Model file for the job. Use its own axes, mm. A direction names the side the tool comes from. Give positions to 0.01 mm unless a question says otherwise; leave off trailing zeros. Loops run counter-clockwise (first coordinate to the right, second up) from the corner with the lowest first, then second, coordinate; pieces in that order, holes last. Notation, with made-up numbers: M 52,36 L 101,36 A32 ccw 101,66 Z; hole C 11,-25 d11. An arc over 180 degrees is marked long. Answer in a Markdown table with one row per item.
Autodesk Inventor part; units mm, degrees
ref_plane "YZ Plane" through (0, 0, 0) normal (1, 0, 0) x (0, 1, 0)
ref_plane "XZ Plane" through (0, 0, 0) normal (0, 1, 0) x (-1, 0, 0)
ref_plane "XY Plane" through (0, 0, 0) normal (0, 0, 1) x (1, 0, 0)
sketch "Sketch1" plane through (0, 0, 0) normal (0, 1, 0) x (-1, 0, 0)
  line L0 (0.5335, -0.6929) -> (33.0335, -0.6929)
  line L1 (33.0335, -0.6929) -> (33.0335, -33.1929)
  line L2 (33.0335, -33.1929) -> (0.5335, -33.1929)
  line L3 (0.5335, -33.1929) -> (0.5335, -0.6929)
  line L4 (-0.7165, 0.5571) -> (34.2835, 0.5571)
  line L5 (34.2835, 0.5571) -> (34.2835, -34.4429)
  line L6 (34.2835, -34.4429) -> (-0.7165, -34.4429)
  line L7 (-0.7165, -34.4429) -> (-0.7165, 0.5571)
  point P0 (0, 0)
  dimension "d0" = 32.5
  dimension "d1" = 32.5
  dimension "d2" = 35
  dimension "d3" = 35
  dimension "d4" = 1.25
  dimension "d5" = 1.25
extrude "Extrusion1" add sketch "Sketch1" along normal blind 3
sketch "Sketch2" plane through (0, 3, 0) normal (0, 1, 0) x (1, 0, 0)
  line L0 (-34.2835, -0.5571) -> (0.7165, -0.5571)
  line L1 (0.7165, -0.5571) -> (0.7165, 34.4429)
  line L2 (-34.2835, -0.5571) -> (0.7165, -0.5571)
  line L3 (0.7165, -0.5571) -> (0.7165, 34.4429)
  line L4 (0.7165, 34.4429) -> (-34.2835, 34.4429)
  line L5 (-34.2835, 34.4429) -> (-34.2835, -0.5571)
  point P0 (0, 0)
extrude "Extrusion2" add sketch "Sketch2" along normal blind 3
sketch "Sketch3" plane through (0, 6, 0) normal (0, 1, 0) x (1, 0, 0)
  line L0 (-21.2835, 12.4429) -> (-12.2835, 12.4429)
  line L1 (-12.2835, 12.4429) -> (-12.2835, 21.4429)
  line L2 (-12.2835, 21.4429) -> (-21.2835, 21.4429)
  line L3 (-21.2835, 21.4429) -> (-21.2835, 12.4429)
  line L4 (-34.2835, 34.4429) -> (-34.2835, -0.5571)
  line L5 (0.7165, 34.4429) -> (-34.2835, 34.4429)
  point P0 (0, 0)
  dimension "d10" = 9
  dimension "d11" = 9
  dimension "d12" = 13
  dimension "d13" = 13
extrude "Extrusion3" cut sketch "Sketch3" against normal blind 3
properties part number "test_camera_seat"
Q1. 3-axis set-ups, long thin cutter, end or side, ignore diameter. For faces 4 (the face through (-17, 5, -21.443)), 5 (the face through (-25, 6, -17)), 6 (the face through (-17, 1, -33.193)): which of +Z, -Z, +X, -X, +Y, -Y reach the whole face in a straight line?
Reported:
| item | result |
|---|---|
| face 4 | +Y, -Y |
| face 5 | +Z, -Z, +X, -X, +Y |
| face 6 | -Y |
Q2. Saw through at D-D (z = -18.5). Give the cut face in (x, y), and give its area (3 significant figures).
Reported:
| item | result |
|---|---|
| outline | M -34.28,0 L -33.03,0 L -33.03,3 L -21.28,3 L -21.28,6 L -34.28,6 Z; M -12.28,3 L -0.53,3 L -0.53,0 L 0.72,0 L 0.72,6 L -12.28,6 Z |
| area | 85.5 mm² |
Q3. Drop a flat-ended pin along its axis: pin 1 (1 mm diameter, centred on x = -23, z = -4, fed in from -Y). Give the stop position or say it passes through.
Reported:
| item | result |
|---|---|
| pin 1 | y = 3 |
Q4. Saw through at A-A (x = -13.5). Give the cut face in (y, z), and give its area (3 significant figures).
Reported:
| item | result |
|---|---|
| outline | M 0,-34.44 L 6,-34.44 L 6,-21.44 L 3,-21.44 L 3,-33.19 L 0,-33.19 Z; M 0,-0.69 L 3,-0.69 L 3,-12.44 L 6,-12.44 L 6,0.56 L 0,0.56 Z |
| area | 85.5 mm² |
Q5. Probe probe 1 along X at (y, z) = (1.55, -21.5); probe 2 along Z at (x, y) = (-14, 0.4); probe 3 along Z at (x, y) = (-15, 4.15). List the from-to ranges inside material, lowest first.
Reported:
| item | result |
|---|---|
| probe 1 | -34.28 to -33.03, -0.53 to 0.72 |
| probe 2 | -34.44 to -33.19, -0.69 to 0.56 |
| probe 3 | -34.44 to -21.44, -12.44 to 0.56 |
Q6. Mould opens along X. For faces 1 (the face through (0.716, 3, -17)), 2 (the face through (-17, 5, -12.443)), 3 (the face through (-15, 0, -34)) say: released by +X, released by -X, zero draft, split by the parting line, or undercut.
Reported:
| item | result |
|---|---|
| face 1 | released by +X |
| face 2 | undercut |
| face 3 | zero draft |
Q7. Saw through at B-B (y = 5.2). Give the cut face in (x, z), and give its area (3 significant figures).
Reported:
| item | result |
|---|---|
| outline | M -34.28,-34.44 L 0.72,-34.44 L 0.72,0.56 L -34.28,0.56 Z; hole M -21.28,-21.44 L -12.28,-21.44 L -12.28,-12.44 L -21.28,-12.44 Z |
| area | 1,140 mm² |
Q8. Saw through at C-C (z = -9.5). Give the cut face in (x, y), and give its area (4 significant figures).
Reported:
| item | result |
|---|---|
| outline | M -34.28,0 L -33.03,0 L -33.03,3 L -0.53,3 L -0.53,0 L 0.72,0 L 0.72,6 L -34.28,6 Z |
| area | 112.5 mm² |
